The listing builds one solid part. Answer for the finished solid, in the listing's coordinates (mm). A direction names the side the tool comes from. Give positions to 0.01 mm unless a question says otherwise; leave off trailing zeros. Write each loop counter-clockwise with the first axis right and the second up, starting at its lowest first coordinate (ties: lowest second). Pieces come first, ordered by that corner, then holes. Notation, with made-up numbers: M 60,61 L 112,61 A8 ccw 112,74 Z; hole C -35.75,-31 d5. An arc over 180 degrees is marked long. Return JSON: item names as keys, results as strings.
from build123d import *

# Parameters (mm, degrees)
BOSS_EXTRUDE1_DEPTH = 15
SKETCH2_W           = 110
SKETCH2_H           = 1
BOSS_EXTRUDE3_DEPTH = 80


with BuildPart() as part:
    # Sketch1 → Boss-Extrude1 (new body)
    with BuildSketch(Plane.XY):
        Polygon((0, 0), (4.913259174, 0), (7.93055075, 8.289940472), (9.992855173, 8.289940472), (13, 0), (17.913259174, 0), (20.93055075, 8.289940472), (22.992855173, 8.289940472), (26, 0), (30.913259174, 0), (33.93055075, 8.289940472), (35.992855173, 8.289940472), (39, 0), (43.913259174, 0), (46.93055075, 8.289940472), (48.992855173, 8.289940472), (52, 0), (56.913259174, 0), (59.93055075, 8.289940472), (61.992855173, 8.289940472), (65, 0), (69.913259174, 0), (72.93055075, 8.289940472), (74.992855173, 8.289940472), (78, 0), (82.913259174, 0), (85.93055075, 8.289940472), (87.992855173, 8.289940472), (91, 0), (95.913259174, 0), (98.93055075, 8.289940472), (100.992855173, 8.289940472), (104, 0), (108.913259174, 0), (111.93055075, 8.289940472), (113.992855173, 8.289940472), (117, 0), (121.913259174, 0), (121.913259174, -10), (0, -10), align=None)
    extrude(amount=BOSS_EXTRUDE1_DEPTH)

    # Sketch2 → Boss-Extrude3 (add)
    with BuildSketch(Plane.XY.offset(15)):
        with Locations((61, -9)):
            Rectangle(SKETCH2_W, SKETCH2_H)
    extrude(amount=BOSS_EXTRUDE3_DEPTH)


solid = part.part
Item 1: A cutting plane is placed at B-B, the plane y = -2.5. Write down the section's boundary in (x, z).
Geometry results:
{"outline": "M 0,0 L 121.91,0 L 121.91,15 L 0,15 Z"}
Item 2: Which of the six approach directions +Z, -Z, +X, -X, +Y, -Y give full straight-line access (tool end or side, diameter ignored) to faces 1 (the flat face through (62, -1, 0)), 2 (the flat face through (41, 0, 7))?
Geometry results:
{"face 1": "-Z, +X, -X, +Y, -Y", "face 2": "+Z, -Z, +Y"}
Item 3: Find the intervals of material crossed by line 1 (Y direction, x = 72.5, z = 79); line 2 (Z direction, x = 30, y = -2.5); line 3 (X direction, y = -9.25, z = 90), in increasing order.
Geometry results:
{"line 1": "y = -9.5 to -8.5", "line 2": "z = 0 to 15", "line 3": "x = 6 to 116"}
Item 4: Determine the mould class of faces 3 (the flat face through (71.4, 4.09, 7.4)), 4 (the flat face through (119, 0, 7)), 5 (the flat face through (0, -5, 7)) for opening direction X: +X half, -X half, draft (parallel to the pull), parting line (faces both ways), or undercut.
Geometry results:
{"face 3": "undercut", "face 4": "draft", "face 5": "-X half"}
Item 5: Given pin 1 Ø4 at (x, z) = (105, 33.5) entering from +Y; pin 2 Ø1.1 at (y, z) = (-9, 54) entering from -X; pin 3 Ø1.5 at (x, z) = (93, 9) entering from +Y, each flat-ended and moving along its own axis, determine where each tip first touches the part or whether it passes through.
Geometry results:
{"pin 1": "stops at y = -8.5", "pin 2": "stops at x = 6", "pin 3": "stops at y = 0"}
Item 6: A cutting plane is placed at A-A, the plane z = 21. Write down the section's boundary in (x, y), plus the area to 3 significant figures.
Geometry results:
{"outline": "M 6,-9.5 L 116,-9.5 L 116,-8.5 L 6,-8.5 Z", "area": "110 mm2"}
